```python
from build123d import *

# Parameters (mm, degrees)
BOSS_EXTRUDE8_DEPTH = 0.17
SKETCH1_W           = 1.5
SKETCH1_H           = 3
SKETCH1_W_2         = 4.66
SKETCH1_H_2         = 1.6
CUT_EXTRUDE1_DEPTH  = 62.727456614


with BuildPart() as part:
    # Sketch13 → Boss-Extrude8 (new body)
    with BuildSketch(Plane.XY):
        with BuildLine():
            Line((-12.5, 60), (4.5, 60))
            ThreePointArc((4.5, 60), (11.571067812, 57.071067812), (14.5, 50))
            Line((14.5, 50), (14.5, -58))
            ThreePointArc((14.5, -58), (13.914213562, -59.414213562), (12.5, -60))
            Line((12.5, -60), (-12.5, -60))
            ThreePointArc((-12.5, -60), (-13.914213562, -59.414213562), (-14.5, -58))
            Line((-14.5, -58), (-14.5, 58))
            ThreePointArc((-14.5, 58), (-13.914213562, 59.414213562), (-12.5, 60))
        make_face()
    extrude(amount=BOSS_EXTRUDE8_DEPTH)

    # Sketch1 → Cut-Extrude1 (cut, through all)
    with BuildSketch(Plane.XY.offset(0.17)):
        with Locations((0, -52.1)):
            Rectangle(SKETCH1_W, SKETCH1_H)
        with Locations((6.41, -8.27)):
            Rectangle(SKETCH1_W_2, SKETCH1_H_2)
        with BuildLine():
            Line((-2.1, 56), (2.1, 56))
            ThreePointArc((2.1, 56), (3.443502884, 55.443502884), (4, 54.1))
            Line((4, 54.1), (4, 38.9))
            ThreePointArc((4, 38.9), (3.443502884, 37.556497116), (2.1, 37))
            Line((2.1, 37), (-2.1, 37))
            ThreePointArc((-2.1, 37), (-3.443502884, 37.556497116), (-4, 38.9))
            Line((-4, 38.9), (-4, 54.1))
            ThreePointArc((-4, 54.1), (-3.443502884, 55.443502884), (-2.1, 56))
        make_face()
        with BuildLine():
            Line((-2.1, 17.931829774), (2.1, 17.931829774))
            ThreePointArc((2.1, 17.931829774), (3.443502884, 17.375332658), (4, 16.031829774))
            Line((4, 16.031829774), (4, 1.6))
            ThreePointArc((4, 1.6), (3.443502884, 0.256497116), (2.1, -0.3))
            Line((2.1, -0.3), (-2.1, -0.3))
            ThreePointArc((-2.1, -0.3), (-3.443502884, 0.256497116), (-4, 1.6))
            Line((-4, 1.6), (-4, 16.031829774))
            ThreePointArc((-4, 16.031829774), (-3.443502884, 17.375332658), (-2.1, 17.931829774))
        make_face()
        with BuildLine():
            Line((2.4, -6.15), (-2.4, -6.15))
            Line((-2.4, -6.15), (-2.4, -29))
            Line((-2.4, -29), (-1.9, -29))
            Line((-1.9, -29), (-8.375, -42.75))
            add(Edge.make_bspline(
                [(-8.375, -42.75), (-8.614001568, -43.20601542), (-8.749703343, -43.736930638), (-8.75, -44.3)],
                knots=[2, 2, 2, 2, 3, 3, 3, 3], degree=3))
            add(Edge.make_bspline(
                [(-8.75, -44.3), (-8.75059415, -45.427724457), (-8.211440188, -46.416320927), (-7.4, -46.97314145)],
                knots=[3, 3, 3, 3, 3.998304655, 3.998304655, 3.998304655, 3.998304655], degree=3))
            Line((-7.4, -46.97314145), (-4.925, -48.85))
            Line((-4.925, -48.85), (-2.6, -49.6))
            Line((-2.6, -49.6), (2.6, -49.6))
            Line((2.6, -49.6), (4.925, -48.85))
            Line((4.925, -48.85), (7.4, -46.97314145))
            add(Edge.make_bspline(
                [(7.4, -46.97314145), (8.211440188, -46.416320927), (8.75059415, -45.427724457), (8.75, -44.3)],
                knots=[3, 3, 3, 3, 3.998304655, 3.998304655, 3.998304655, 3.998304655], degree=3))
            add(Edge.make_bspline(
                [(8.75, -44.3), (8.749703343, -43.736930638), (8.614001568, -43.20601542), (8.375, -42.75)],
                knots=[2, 2, 2, 2, 3, 3, 3, 3], degree=3))
            Line((8.375, -42.75), (1.9, -29))
            Line((1.9, -29), (2.4, -29))
            Line((2.4, -29), (2.4, -6.15))
        make_face()
    extrude(amount=-CUT_EXTRUDE1_DEPTH, mode=Mode.SUBTRACT)


solid = part.part
```
Design review of the part built by this model. Coordinates are the model's own, in mm. Coordinates: 2 decimals unless noted, no trailing zeros. Loops run counter-clockwise (first coordinate to the right, second up) from the corner with the lowest first, then second, coordinate; pieces in that order, holes last. Notation, with made-up numbers: (45, -11.5) - (59, -11.5) arc R26 ccw to (59, 2.5) - close; hole circle Ø7 at (87, 78.5). An arc over 180 degrees is marked (long way). Use CSV: the item, a comma, the result in double quotes. Start each with the question number.
1) Wall thickness on L1, parallel to Y at x = -1.25, z = 0.1; L2, parallel to Y at x = -2.5, z = 0.1; L3, parallel to X at y = 15.5, z = 0.1: over which ranges is each line inside the solid? List them lowest first. Write a range as from..to.
2) Consider section A-A on y = 41. Write out the cut boundary in (x, z).
3) Consider section C-C on y = -13.5. Write out the cut boundary in (x, z).
4) Consider section B-B on z = 0.1. Give the number of separate pieces and of enclosed holes in the cut face, then the cut area to 3 significant figures.
Geometry says:
1,L1,"-60..-49.6, -6.15..-0.3, 17.93..37, 56..60"
1,L2,"-60..-49.6, -30.27..-0.26, 17.89..37.04, 55.96..60"
1,L3,"-14.5..-4, 4..14.5"
2,outline,"(-14.5, 0) - (-4, 0) - (-4, 0.17) - (-14.5, 0.17) - close; (4, 0) - (14.5, 0) - (14.5, 0.17) - (4, 0.17) - close"
3,outline,"(-14.5, 0) - (-2.4, 0) - (-2.4, 0.17) - (-14.5, 0.17) - close; (2.4, 0) - (14.5, 0) - (14.5, 0.17) - (2.4, 0.17) - close"
4,separate pieces,"1"
4,enclosed holes,"5"
4,area,"2,800 mm^2"
